```python
from build123d import *

# Parameters (mm, degrees)
SKETCH1_W           = 12
SKETCH1_H           = 17
BOSS_EXTRUDE1_DEPTH = 11
SKETCH2_W           = 8.2
SKETCH2_H           = 8.2
CUT_EXTRUDE1_DEPTH  = 15
SKETCH3_W           = 6
SKETCH3_H           = 3
BOSS_EXTRUDE2_DEPTH = 15
CHAMFER1_SIZE       = 1.120110988
CHAMFER1_SIZE2      = 1.260754717
CHAMFER2_SIZE       = 1.260754717
CHAMFER2_SIZE2      = 1.120110988


with BuildPart() as part:
    # Sketch1 → Boss-Extrude1 (new body)
    with BuildSketch(Plane(origin=(0, 0, -5.5), x_dir=(-1, 0, 0), z_dir=(0, 0, -1))):
        with Locations((0, 8.5)):
            Rectangle(SKETCH1_W, SKETCH1_H)
    extrude(amount=-BOSS_EXTRUDE1_DEPTH)

    # Sketch2 → Cut-Extrude1 (cut)
    with BuildSketch(Plane.XZ):
        Rectangle(SKETCH2_W, SKETCH2_H)
    extrude(amount=-CUT_EXTRUDE1_DEPTH, mode=Mode.SUBTRACT)

    # Sketch3 → Boss-Extrude2 (add)
    with BuildSketch(Plane.XZ.offset(-15)):
        Rectangle(SKETCH3_W, SKETCH3_H)
    extrude(amount=BOSS_EXTRUDE2_DEPTH)

    # Chamfer1
    chamfer1_edges = [part.edges().sort_by_distance(p)[0] for p in [
        (4.1, 7.5, 4.1),
    ]]
    chamfer1_side = [part.faces().sort_by_distance(p)[0] for p in [
        (0, 7.5, 4.1),
    ]]
    chamfer(chamfer1_edges, length=CHAMFER1_SIZE, length2=CHAMFER1_SIZE2, reference=chamfer1_side[0])

    # Chamfer2
    chamfer2_edges = [part.edges().sort_by_distance(p)[0] for p in [
        (-4.1, 7.5, 4.1),
    ]]
    chamfer2_side = [part.faces().sort_by_distance(p)[0] for p in [
        (-4.1, 7.5, 0),
    ]]
    chamfer(chamfer2_edges, length=CHAMFER2_SIZE, length2=CHAMFER2_SIZE2, reference=chamfer2_side[0])


solid = part.part
```
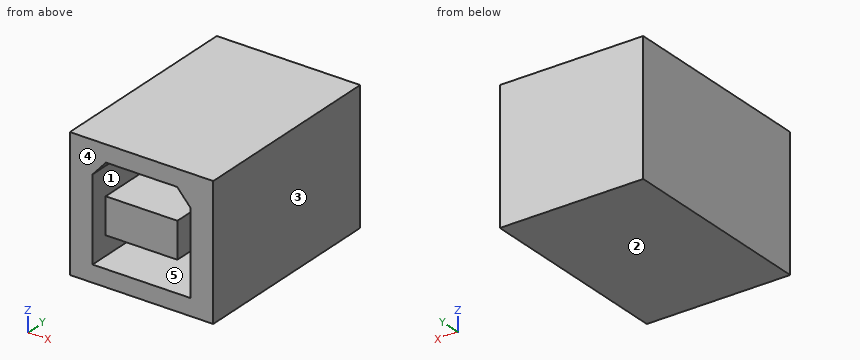
Source: CAD feature listing. Evaluate the final solid. Frame: model axes, mm. Face numbers are marked on the shaded views. A direction names the side the tool comes from. Round coordinates to 2 decimals unless told otherwise and drop trailing zeros. Write each loop counter-clockwise with the first axis right and the second up, starting at its lowest first coordinate (ties: lowest second). Pieces come first, ordered by that corner, then holes. Notation, with made-up numbers: M 55.25,43.5 L 82.25,43.5 A17 cw 82.25,64.5 Z; hole C 5.25,30.25 d6. An arc over 180 degrees is marked long. Answer as a JSON object with one key per item and string values. Group by question number.
(1) Section query D-D on x = 3.5. Output: boundary loops of the cut face in (y, z), then the cut area to 3 significant figures.
(2) Section query A-A on y = 8.25. Output: boundary loops of the cut face in (x, z).
(3) Mould query, pull axis X, two halves, no side actions, for the marked faces 1, 2 and 3. Classes: +X half, -X half, draft (parallel to the pull), parting line (faces both ways), or undercut.
(4) Ray query, line 1 (Z direction, x = -1.5, y = 11); line 2 (X direction, y = 5.25, z = 0.5); line 3 (Y direction, x = 0.25, z = -3.25). Return the intervals inside material, ascending. Write a range as [from, to].
(5) Section query C-C on z = 2.25. Output: boundary loops of the cut face in (x, y), then the cut area to 3 significant figures.
(6) Reachability of the marked faces 4 and 5 from +Z, -Z, +X, -X, +Y, -Y: full face, straight path, thin tool, end or side. Return the list, or none.
(7) Section query B-B on x = 1.5. Output: boundary loops of the cut face in (y, z).
Computed values:
{
 "1": {"outline": "M 0,-5.5 L 17,-5.5 L 17,5.5 L 0,5.5 L 0,3.51 L 15,3.51 L 15,-4.1 L 0,-4.1 Z", "area": "72.8 mm^2"},
 "2": {"outline": "M -6,-5.5 L 6,-5.5 L 6,5.5 L -6,5.5 Z; M -3,-1.5 L 3,-1.5 L 3,1.5 L -3,1.5 Z; hole M -4.1,-4.1 L 4.1,-4.1 L 4.1,2.84 L 2.98,4.1 L -2.98,4.1 L -4.1,2.84 Z"},
 "3": {"face 1": "undercut", "face 2": "draft", "face 3": "+X half"},
 "4": {"line 1": "[-5.5, -4.1], [-1.5, 1.5], [4.1, 5.5]", "line 2": "[-6, -4.1], [-3, 3], [4.1, 6]", "line 3": "[15, 17]"},
 "5": {"outline": "M -6,0 L -4.1,0 L -4.1,15 L 4.1,15 L 4.1,0 L 6,0 L 6,17 L -6,17 Z", "area": "81.0 mm^2"},
 "6": {"face 4": "+Z, -Z, +X, -X, -Y", "face 5": "-Y"},
 "7": {"outline": "M 0,-5.5 L 17,-5.5 L 17,5.5 L 0,5.5 L 0,4.1 L 15,4.1 L 15,1.5 L 0,1.5 L 0,-1.5 L 15,-1.5 L 15,-4.1 L 0,-4.1 Z"}
}
